Geometry: final body of the model. Coordinates: model frame, mm. Face numbers are marked on the shaded views. A direction names the side the tool comes from. Give positions to 0.01 mm unless a question says otherwise; leave off trailing zeros. Loops run counter-clockwise (first coordinate to the right, second up) from the corner with the lowest first, then second, coordinate; pieces in that order, holes last.
from build123d import *

# Parameters (mm, degrees)
SKETCH1_R         = 14.5
BODY_DEPTH        = 2
SKETCH2_R         = 1.5
FIXHOLES_DEPTH    = 2
SKETCH3_R         = 11.5
BODY2_DEPTH       = 3
SKETCH5_W         = 11
SKETCH5_H         = 11
WINDOW_HOLE_DEPTH = 12
SKETCH7_W         = 13
SKETCH7_H         = 13
WINDOW_DEPTH      = 0.25
WINDOW_FILLET_R   = 1


with BuildPart() as part:
    # Sketch1 → Body (new body)
    with BuildSketch(Plane(origin=(0, 0, 0), x_dir=(1, 0, 0), z_dir=(0, 1, 0))):
        Circle(SKETCH1_R)
    extrude(amount=BODY_DEPTH)

    # Sketch2 → FixHoles (add)
    with BuildSketch(Plane.XZ):
        with Locations((0, 11)):
            Circle(SKETCH2_R)
        with Locations((0, -11)):
            Circle(SKETCH2_R)
    extrude(amount=FIXHOLES_DEPTH)

    # Sketch3 → Body2 (add)
    with BuildSketch(Plane(origin=(0, 2, 0), x_dir=(1, 0, 0), z_dir=(0, 1, 0))):
        Circle(SKETCH3_R)
    extrude(amount=BODY2_DEPTH)

    # Sketch5 → Window_hole (cut)
    with BuildSketch(Plane.XZ):
        Rectangle(SKETCH5_W, SKETCH5_H)
    extrude(amount=-WINDOW_HOLE_DEPTH, mode=Mode.SUBTRACT)

    # Sketch6 → Objective_cut (revolve, cut)
    with BuildSketch(Plane.XY):
        Polygon((-5.5, 5), (-10.5, 5), (-5.5, 0.5), align=None)
    revolve(axis=Axis((0, 7.375311512, 0), (0, -1, 0)), mode=Mode.SUBTRACT)

    # Sketch7 → Window (cut)
    with BuildSketch(Plane.XZ):
        Rectangle(SKETCH7_W, SKETCH7_H)
    extrude(amount=-WINDOW_DEPTH, mode=Mode.SUBTRACT)

    # Window_Fillet
    window_fillet_edges = [part.edges().sort_by_distance(p)[0] for p in [
        (-5.5, 1.400178567, 5.5),
        (5.5, 1.400178567, 5.5),
        (5.5, 1.400178567, -5.5),
        (-5.5, 1.400178567, -5.5),
    ]]
    fillet(window_fillet_edges, radius=WINDOW_FILLET_R)


solid = part.part
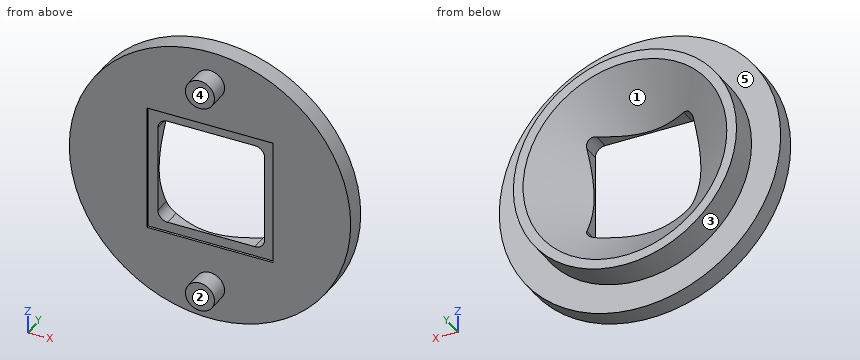
Item 1: Draft query along X for the marked faces 1, 2 and 3. Return one class per face: +X half, -X half, draft (parallel to the pull), parting line (faces both ways), or undercut.
Values follow:
face 1: undercut
face 2: draft
face 3: parting line
Item 2: Section query B-B on y = 1.25. Return loops of the section in (x, z).
Values follow:
outline: circle Ø29 at (0, 0); hole (-5.5, -4.5) arc R1 ccw to (-4.5, -5.5) - (-3.14, -5.5) arc R6.33 ccw to (3.14, -5.5) - (4.5, -5.5) arc R1 ccw to (5.5, -4.5) - (5.5, -3.14) arc R6.33 ccw to (5.5, 3.14) - (5.5, 4.5) arc R1 ccw to (4.5, 5.5) - (3.14, 5.5) arc R6.33 ccw to (-3.14, 5.5) - (-4.5, 5.5) arc R1 ccw to (-5.5, 4.5) - (-5.5, 3.14) arc R6.33 ccw to (-5.5, -3.14) - close
Item 3: Set-up query: the marked faces 4 and 5. Return all of +Z, -Z, +X, -X, +Y, -Y with unobstructed straight access to the full face (end or side cutting, diameter ignored); none if empty.
Values follow:
face 4: +Z, -Z, +X, -X, -Y
face 5: +Y
Item 4: Section query D-D on z = 12. Return loops of the section in (x, y).
Values follow:
outline: (-8.14, 0) - (-1.12, 0) - (-1.12, -2) - (1.12, -2) - (1.12, 0) - (8.14, 0) - (8.14, 2) - (-8.14, 2) - close
Item 5: Section query A-A on x = 0. Return loops of the section in (y, z).
Values follow:
outline: (-2, -12.5) - (0, -12.5) - (0, -14.5) - (2, -14.5) - (2, -11.5) - (5, -11.5) - (5, -10.5) - (0.5, -5.5) - (0.25, -5.5) - (0.25, -6.5) - (0, -6.5) - (0, -9.5) - (-2, -9.5) - close; (-2, 9.5) - (0, 9.5) - (0, 6.5) - (0.25, 6.5) - (0.25, 5.5) - (0.5, 5.5) - (5, 10.5) - (5, 11.5) - (2, 11.5) - (2, 14.5) - (0, 14.5) - (0, 12.5) - (-2, 12.5) - close
Item 6: Section query C-C on y = -1. Return loops of the section in (x, z), plus the area to 3 significant figures.
Values follow:
outline: circle Ø3 at (0, -11); circle Ø3 at (0, 11)
area: 14.1 mm2
Item 7: Ray query, probe 1 along Y at (x, z) = (13, -0.5); probe 2 along Y at (x, z) = (4.5, -10.25); probe 3 along Z at (x, y) = (4.5, 1.75). Return the intervals inside material, ascending.
Values follow:
probe 1: y = 0 to 2
probe 2: y = 0 to 5
probe 3: z = -13.78 to -5.5, 5.5 to 13.78
Item 8: Pin query (flat end, axial travel): pin 1 (4 mm diameter, centred on x = -9, z = 11, fed in from -Y); pin 2 (1.5 mm diameter, centred on x = -5.5, z = -1, fed in from +Y); pin 3 (1.4 mm diameter, centred on x = -1, y = 1.5, fed in from -Z). Return the tip coordinate at first contact, or that it passes through.
Values follow:
pin 1: stops at y = 0
pin 2: stops at y = 1.26
pin 3: stops at z = -14.5
